Source: CAD feature listing. Evaluate the final solid. Frame: model axes, mm. A direction names the side the tool comes from. Give positions to 0.01 mm unless a question says otherwise; leave off trailing zeros. Write each loop counter-clockwise with the first axis right and the second up, starting at its lowest first coordinate (ties: lowest second). Pieces come first, ordered by that corner, then holes.
```python
from build123d import *

# Parameters (mm, degrees)
SKETCH1_W           = 183.739955438
SKETCH1_H           = 42.541825
SKETCH1_R           = 2.2479
BOSS_EXTRUDE1_DEPTH = 9.525
SKETCH1_5_R         = 2.2479
CUT_EXTRUDE1_DEPTH  = 6.35
CUT_EXTRUDE2_DEPTH  = 181.771443479
CUT_EXTRUDE3_DEPTH  = 2.54


with BuildPart() as part:
    # Sketch1 → Boss-Extrude1 (new body)
    with BuildSketch(Plane(origin=(0, 0, 0), x_dir=(1, 0, 0), z_dir=(0, 1, 0))):
        with Locations((83.566, 21.2709125)):
            Rectangle(SKETCH1_W, SKETCH1_H)
        with Locations(Location((45.72, 38.1, 0), (0, 0, 270))):
            Circle(SKETCH1_R, mode=Mode.SUBTRACT)
        with Locations(Location((38.1, 38.1, 0), (0, 0, 270))):
            Circle(SKETCH1_R, mode=Mode.SUBTRACT)
        with Locations(Location((30.48, 38.1, 0), (0, 0, 270))):
            Circle(SKETCH1_R, mode=Mode.SUBTRACT)
        with Locations(Location((22.86, 38.1, 0), (0, 0, 270))):
            Circle(SKETCH1_R, mode=Mode.SUBTRACT)
        with Locations(Location((15.24, 38.1, 0), (0, 0, 270))):
            Circle(SKETCH1_R, mode=Mode.SUBTRACT)
        with Locations(Location((7.62, 38.1, 0), (0, 0, 270))):
            Circle(SKETCH1_R, mode=Mode.SUBTRACT)
        with Locations(Location((0, 38.1, 0), (0, 0, 270))):
            Circle(SKETCH1_R, mode=Mode.SUBTRACT)
        with Locations(Location((53.34, 38.1, 0), (0, 0, 270))):
            Circle(SKETCH1_R, mode=Mode.SUBTRACT)
        with Locations(Location((142.748, 38.1, 0), (0, 0, 270))):
            Circle(SKETCH1_R, mode=Mode.SUBTRACT)
        with Locations(Location((134.62, 38.1, 0), (0, 0, 270))):
            Circle(SKETCH1_R, mode=Mode.SUBTRACT)
        with Locations(Location((126.492, 38.1, 0), (0, 0, 270))):
            Circle(SKETCH1_R, mode=Mode.SUBTRACT)
        with Locations(Location((118.364, 38.1, 0), (0, 0, 270))):
            Circle(SKETCH1_R, mode=Mode.SUBTRACT)
        with Locations(Location((110.236, 38.1, 0), (0, 0, 270))):
            Circle(SKETCH1_R, mode=Mode.SUBTRACT)
        with Locations(Location((150.876, 38.1, 0), (0, 0, 270))):
            Circle(SKETCH1_R, mode=Mode.SUBTRACT)
        with Locations(Location((159.004, 38.1, 0), (0, 0, 270))):
            Circle(SKETCH1_R, mode=Mode.SUBTRACT)
        with Locations(Location((167.132, 38.1, 0), (0, 0, 270))):
            Circle(SKETCH1_R, mode=Mode.SUBTRACT)
    extrude(amount=-BOSS_EXTRUDE1_DEPTH)

    # Sketch1<5> → Cut-Extrude1 (cut)
    # profile 1 of 2: a face of its own
    with BuildSketch(Plane(origin=(0, 0, 0), x_dir=(1, 0, 0), z_dir=(0, 1, 0))):
        Polygon((-5.128977719, 38.1), (-2.564488859, 33.658175), (2.564488859, 33.658175), (3.81, 35.815463577), (5.055511141, 33.658175), (10.184488859, 33.658175), (11.43, 35.815463577), (12.675511141, 33.658175), (17.804488859, 33.658175), (19.05, 35.815463577), (20.295511141, 33.658175), (25.424488859, 33.658175), (26.67, 35.815463577), (27.915511141, 33.658175), (33.044488859, 33.658175), (34.29, 35.815463577), (35.535511141, 33.658175), (40.664488859, 33.658175), (41.91, 35.815463577), (43.155511141, 33.658175), (48.284488859, 33.658175), (49.53, 35.815463577), (50.775511141, 33.658175), (55.904488859, 33.658175), (58.468977719, 38.1), (58.468977719, 42.541825), (-5.128977719, 42.541825), align=None)
        with Locations((0, 38.1)):
            Circle(SKETCH1_5_R, mode=Mode.SUBTRACT)
        with Locations((7.62, 38.1)):
            Circle(SKETCH1_5_R, mode=Mode.SUBTRACT)
        with Locations((15.24, 38.1)):
            Circle(SKETCH1_5_R, mode=Mode.SUBTRACT)
        with Locations((22.86, 38.1)):
            Circle(SKETCH1_5_R, mode=Mode.SUBTRACT)
        with Locations((30.48, 38.1)):
            Circle(SKETCH1_5_R, mode=Mode.SUBTRACT)
        with Locations((38.1, 38.1)):
            Circle(SKETCH1_5_R, mode=Mode.SUBTRACT)
        with Locations((45.72, 38.1)):
            Circle(SKETCH1_5_R, mode=Mode.SUBTRACT)
        with Locations((53.34, 38.1)):
            Circle(SKETCH1_5_R, mode=Mode.SUBTRACT)
    # profile 2 of 2: a face of its own
    with BuildSketch(Plane(origin=(0, 0, 0), x_dir=(1, 0, 0), z_dir=(0, 1, 0))):
        Polygon((164.567511141, 33.658175), (169.696488859, 33.658175), (172.260977719, 38.1), (172.260977719, 42.541825), (105.107022281, 42.541825), (105.107022281, 38.1), (107.671511141, 33.658175), (112.800488859, 33.658175), (114.3, 36.255404482), (115.799511141, 33.658175), (120.928488859, 33.658175), (122.428, 36.255404482), (123.927511141, 33.658175), (129.056488859, 33.658175), (130.556, 36.255404482), (132.055511141, 33.658175), (137.184488859, 33.658175), (138.684, 36.255404482), (140.183511141, 33.658175), (145.312488859, 33.658175), (146.812, 36.255404482), (148.311511141, 33.658175), (153.440488859, 33.658175), (154.94, 36.255404482), (156.439511141, 33.658175), (161.568488859, 33.658175), (163.068, 36.255404482), align=None)
        with Locations((110.236, 38.1)):
            Circle(SKETCH1_5_R, mode=Mode.SUBTRACT)
        with Locations((118.364, 38.1)):
            Circle(SKETCH1_5_R, mode=Mode.SUBTRACT)
        with Locations((126.492, 38.1)):
            Circle(SKETCH1_5_R, mode=Mode.SUBTRACT)
        with Locations((134.62, 38.1)):
            Circle(SKETCH1_5_R, mode=Mode.SUBTRACT)
        with Locations((142.748, 38.1)):
            Circle(SKETCH1_5_R, mode=Mode.SUBTRACT)
        with Locations((150.876, 38.1)):
            Circle(SKETCH1_5_R, mode=Mode.SUBTRACT)
        with Locations((159.004, 38.1)):
            Circle(SKETCH1_5_R, mode=Mode.SUBTRACT)
        with Locations((167.132, 38.1)):
            Circle(SKETCH1_5_R, mode=Mode.SUBTRACT)
    extrude(amount=-CUT_EXTRUDE1_DEPTH, mode=Mode.SUBTRACT)

    # Mirror1: part across plane


with BuildPart() as part_1:
    add(part.part)
    add(part.part.mirror(Plane.XY))

    # Sketch2 → Cut-Extrude2 (cut, through all)
    with BuildSketch(Plane(origin=(0, 0, 0), x_dir=(1, 0, 0), z_dir=(0, 1, 0))):
        with BuildLine():
            Line((142.748, -19), (134.62, -19))
            ThreePointArc((134.62, -19), (115.62, 0), (134.62, 19))
            Line((134.62, 19), (142.748, 19))
            ThreePointArc((142.748, 19), (161.748, 0), (142.748, -19))
        make_face()
        with BuildLine():
            Line((28.956, -19), (24.384, -19))
            ThreePointArc((24.384, -19), (5.384, 0), (24.384, 19))
            Line((24.384, 19), (28.956, 19))
            ThreePointArc((28.956, 19), (47.956, 0), (28.956, -19))
        make_face()
    extrude(amount=-CUT_EXTRUDE2_DEPTH, mode=Mode.SUBTRACT)

    # Sketch4 → Cut-Extrude3 (cut)
    with BuildSketch(Plane(origin=(0, 0, 0), x_dir=(1, 0, 0), z_dir=(0, 1, 0))):
        Polygon((75.438, 26.463302372), (81.788, 37.461825), (88.138, 26.463302372), align=None)
    extrude(amount=-CUT_EXTRUDE3_DEPTH, mode=Mode.SUBTRACT)


solid = part_1.part
```
1. Line query: probe 1 along X at (y, z) = (-4.75, -1); probe 2 along Z at (x, y) = (134.62, -8.4); probe 3 along X at (y, z) = (-2, 9). Output: solid intervals per line, ascending.
2. Access query for faces 3 (the flat face through (106.37, -3.13, -35.91)), 4 (the flat face through (139, -5, 19)), 5 (the flat face through (84.92, -1.25, -32.04)), 6 (the flat face through (172.261, -3, 40)). Directions: +Z, -Z, +X, -X, +Y, -Y. A direction counts if a zero-diameter tool reaches every point of the face in a straight line with its end or side. Return the directions, or none.
3. Pin query (flat end, axial travel): P1, Ø8, axis at x = 128, z = 9, coming from the +Y side; P2, Ø1.5, axis at x = 142.5, y = -4, coming from the -Z side; P3, Ø2.5, axis at x = 15.5, y = -3.5, coming from the +Z side; P4, Ø5.5, axis at x = 119.5, y = -2.5, coming from the -Z side. Return the tip coordinate at first contact, or that it passes through.
4. Pull-direction query (X, two-part tool) for faces 1 (the flat face through (82, -9.525, 1)), 2 (the flat face through (138, -6.35, 38)); classes: pulls with the +X half, pulls with the -X half, needs draft (parallel to the pull), parting line crosses it, or undercut.
5. Section query A-A (z = 0). Return loops of the section in (x, y) (3 decimals).
6. Section query B-B (x = 0). Return loops of the section in (y, z) (3 decimals), plus the area to 3 significant figures.
7. Section query C-C (z = 9). Return loops of the section in (x, y) (3 decimals).
The answers:
1. probe 1: x = -8.3 to 5.41, 47.93 to 115.65, 161.72 to 175.44
1. probe 2: z = -42.54 to -40.35, -35.85 to -19, 19 to 35.85, 40.35 to 42.54
1. probe 3: x = -8.3 to 7.65, 45.69 to 117.89, 159.48 to 175.44
2. face 3: -Z, +Y
2. face 4: +Y, -Y
2. face 5: +Y
2. face 6: +Z, +Y
3. P1: passes through
3. P2: stops at z = -33.66
3. P3: stops at z = 33.66
3. P4: stops at z = -35.95
4. face 1: needs draft
4. face 2: undercut
5. outline: (-8.304, -9.525) - (5.384, -9.525) - (5.384, 0) - (-8.304, 0) - close; (47.956, -9.525) - (115.62, -9.525) - (115.62, 0) - (47.956, 0) - close; (161.748, -9.525) - (175.436, -9.525) - (175.436, 0) - (161.748, 0) - close
6. outline: (-9.525, -42.542) - (-6.35, -42.542) - (-6.35, -40.348) - (-9.525, -40.348) - close; (-9.525, -35.852) - (-6.35, -35.852) - (-6.35, -33.658) - (0, -33.658) - (0, 33.658) - (-6.35, 33.658) - (-6.35, 35.852) - (-9.525, 35.852) - close; (-9.525, 40.348) - (-6.35, 40.348) - (-6.35, 42.542) - (-9.525, 42.542) - close
6. area: 669 mm2
7. outline: (-8.304, -9.525) - (7.651, -9.525) - (7.651, 0) - (-8.304, 0) - close; (45.689, -9.525) - (117.887, -9.525) - (117.887, 0) - (45.689, 0) - close; (159.481, -9.525) - (175.436, -9.525) - (175.436, 0) - (159.481, 0) - close
